```python
from build123d import *

# Parameters (mm, degrees)
BOSS_EXTRUDE1_DEPTH      = 380
BOSS_EXTRUDE1_DEPTH_BACK = 380


with BuildPart() as part:
    # Sketch1 → Boss-Extrude1 (new, two sides: drawn at the far end of the back side and taken through both)
    with BuildSketch(Plane(origin=(0, 0, 0), x_dir=(1, 0, 0), z_dir=(0, 1, 0)).offset(-BOSS_EXTRUDE1_DEPTH_BACK)):
        with BuildLine():
            Line((-61.712368752, -98.334403464), (-14.947893024, 461.249197402))
            ThreePointArc((-14.947893024, 461.249197402), (0, 475), (14.947893024, 461.249197402))
            Line((14.947893024, 461.249197402), (61.712368752, -98.334403464))
            ThreePointArc((61.712368752, -98.334403464), (56.501082654, -113.540459174), (41.78184472, -120))
            Line((41.78184472, -120), (-41.78184472, -120))
            ThreePointArc((-41.78184472, -120), (-56.501082654, -113.540459174), (-61.712368752, -98.334403464))
        make_face()
    extrude(amount=BOSS_EXTRUDE1_DEPTH + BOSS_EXTRUDE1_DEPTH_BACK)


solid = part.part
```
Model file for the job. Use its own axes, mm. Give positions to 0.01 mm unless a question says otherwise; leave off trailing zeros. Write each loop counter-clockwise with the first axis right and the second up, starting at its lowest first coordinate (ties: lowest second). Pieces come first, ordered by that corner, then holes. Notation, with made-up numbers: M 89,54.25 L 147,54.25 A20 ccw 147,71.25 Z; hole C 5,-11.5 d10. An arc over 180 degrees is marked long. Use a Markdown table: item, result.
1) Cut at A-A (y = -134.5). List the corners of the cut face in (x, z).
Responses:
| item | result |
|---|---|
| outline | M -61.71,98.33 L -14.95,-461.25 A15 ccw 14.95,-461.25 L 61.71,98.33 A20 ccw 41.78,120 L -41.78,120 A20 ccw Z |
2) Drill centre lines: line 1 (Z direction, x = 1, y = -282); line 2 (X direction, y = 335.5, z = -190.5); line 3 (X direction, y = -112, z = 19.5). Where is each one in solid material? Low to high. Write a range as from..to.
Responses:
| item | result |
|---|---|
| line 1 | z = -474.97..120 |
| line 2 | x = -37.57..37.57 |
| line 3 | x = -55.12..55.12 |
3) Pin check, flat tips, straight feed: pin 1 (5 mm diameter, centred on y = -120.5, z = -343, fed in from +X); pin 2 (12 mm diameter, centred on y = 19, z = -382.5, fed in from -X); pin 3 (10 mm diameter, centred on y = -0.5, z = 4, fed in from +X). Stop position of each tip, or through.
Responses:
| item | result |
|---|---|
| pin 1 | stops at x = 25.04 |
| pin 2 | stops at x = -22.03 |
| pin 3 | stops at x = 54.25 |
4) Cut at B-B (z = -158.5). List the corners of the cut face in (x, y), and give its area (3 significant figures).
Responses:
| item | result |
|---|---|
| outline | M -40.25,-380 L 40.25,-380 L 40.25,380 L -40.25,380 Z |
| area | 61,200 mm2 |
5) Cut at C-C (z = -41). List the corners of the cut face in (x, y).
Responses:
| item | result |
|---|---|
| outline | M -50.07,-380 L 50.07,-380 L 50.07,380 L -50.07,380 Z |
